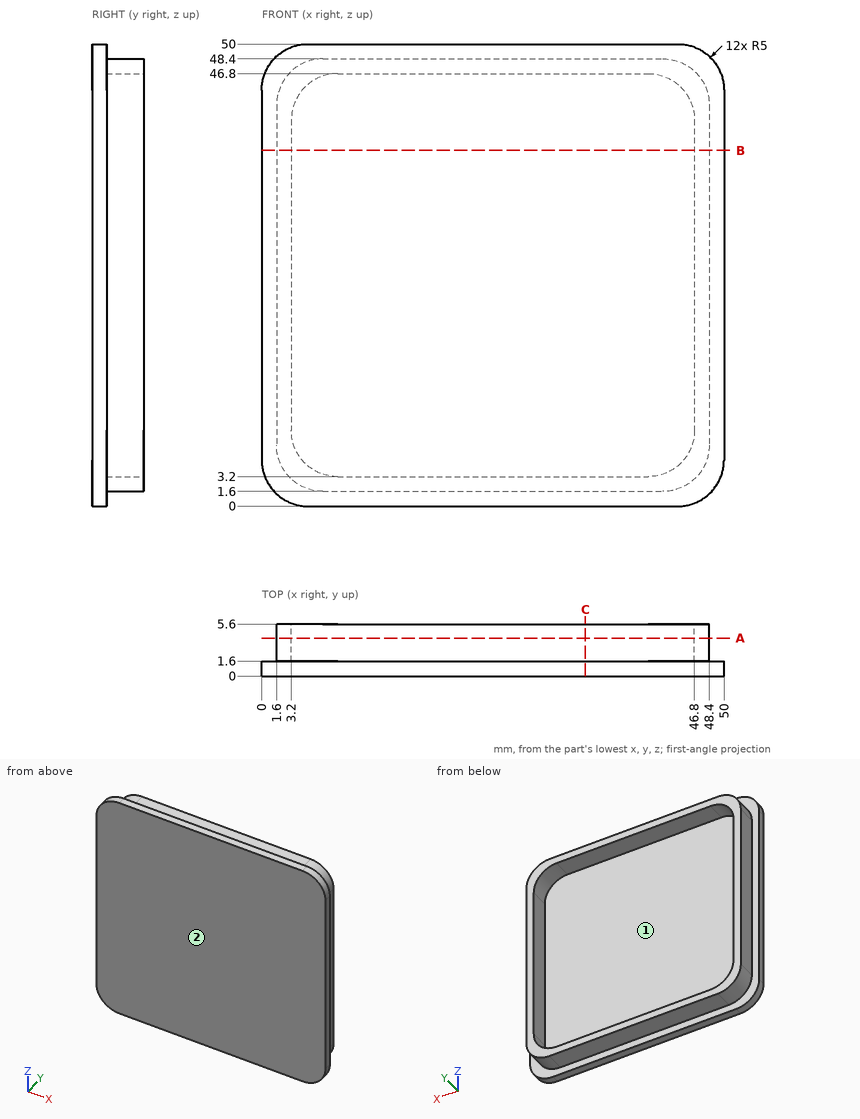
Part print with two shaded views. Sizes in mm from the minimum x, y, z corner. Round coordinates to 2 decimals unless told otherwise and drop trailing zeros. Order: outer loops, then holes, each group sorted by start corner. A loop starts at its lowest first (then second) coordinate and runs counter-clockwise, first axis right, second up. Notation, with made-up numbers: M -28,6 L -1,6 A15 cw -1,24 Z; hole C 20.5,31.25 d5. An arc over 180 degrees is marked long. Put each result on its own line as item: value. Start each with the question number.
1. Two-plate mould, pull along X, no slides. Class the marked faces 1 and 2: +X half, -X half, draft (parallel to the pull), parting line (faces both ways), or undercut.
2. Drill centre lines: probe 1 along X at (y, z) = (3.25, 12.5); probe 2 along Y at (x, z) = (10, 44). Where is each one in solid material? Low to high. Write a range as [from, to].
3. Slice it at A-A on y = 4.1. List the corners of the cut face in (x, z), then the cut area to 3 significant figures.
4. Slice it at B-B on z = 38.5. List the corners of the cut face in (x, y), then the cut area to 3 significant figures.
5. Slice it at C-C on x = 35. List the corners of the cut face in (y, z), then the cut area to 3 significant figures.
6. Drop flat-ended pins along their axis: pin 1 (1.5 mm diameter, centred on x = 24, z = 32.5, fed in from +Y); pin 2 (1.2 mm diameter, centred on x = 30.5, y = 3, fed in from +Z); pin 3 (1.2 mm diameter, centred on y = 3, z = 25, fed in from +X). Give the stop position or say it passes through.
Findings:
1. face 1: undercut
1. face 2: draft
2. probe 1: [1.6, 3.2], [46.8, 48.4]
2. probe 2: [0, 1.6]
3. outline: M 1.6,6.6 A5 ccw 6.6,1.6 L 43.4,1.6 A5 ccw 48.4,6.6 L 48.4,43.4 A5 ccw 43.4,48.4 L 6.6,48.4 A5 ccw 1.6,43.4 Z; hole M 3.2,8.2 A5 ccw 8.2,3.2 L 41.8,3.2 A5 ccw 46.8,8.2 L 46.8,41.8 A5 ccw 41.8,46.8 L 8.2,46.8 A5 ccw 3.2,41.8 Z
3. area: 289 mm2
4. outline: M 0,0 L 50,0 L 50,1.6 L 48.4,1.6 L 48.4,5.6 L 46.8,5.6 L 46.8,1.6 L 3.2,1.6 L 3.2,5.6 L 1.6,5.6 L 1.6,1.6 L 0,1.6 Z
4. area: 92.8 mm2
5. outline: M 0,0 L 1.6,0 L 1.6,1.6 L 5.6,1.6 L 5.6,3.2 L 1.6,3.2 L 1.6,46.8 L 5.6,46.8 L 5.6,48.4 L 1.6,48.4 L 1.6,50 L 0,50 Z
5. area: 92.8 mm2
6. pin 1: y = 1.6
6. pin 2: z = 48.4
6. pin 3: x = 48.4
